```python
from build123d import *

# Parameters (mm, degrees)
BOSS_EXTRUDE1_DEPTH = 2
BOSS_EXTRUDE2_DEPTH = 1
SKETCH3_R           = 3.5
BOSS_EXTRUDE4_DEPTH = 11
SKETCH4_R           = 12.25
BOSS_EXTRUDE5_DEPTH = 6.5


with BuildPart() as part:
    # Sketch1 → Boss-Extrude1 (new body)
    with BuildSketch(Plane(origin=(0, 0, 0), x_dir=(1, 0, 0), z_dir=(0, 1, 0))):
        with BuildLine():
            Line((-14, 10), (-7.665507159, 10))
            ThreePointArc((-7.665507159, 10), (12.6, 0), (-7.665507159, -10))
            Line((-7.665507159, -10), (-14, -10))
            Line((-14, -10), (-14, 10))
        make_face()
    extrude(amount=BOSS_EXTRUDE1_DEPTH)

    # Sketch2 → Boss-Extrude2 (add)
    with BuildSketch(Plane.XY.offset(10)):
        with BuildLine():
            Line((0, 2), (-13.412192981, 19.716181289))
            ThreePointArc((-13.412192981, 19.716181289), (-19.325951381, 20.85226559), (-21.074450498, 15.089802853))
            Line((-21.074450498, 15.089802853), (-14, 0))
            Line((-14, 0), (0, 0))
            Line((0, 0), (0, 2))
        make_face()
    boss_extrude2 = extrude(amount=BOSS_EXTRUDE2_DEPTH)

    # Sketch3 → Boss-Extrude4 (add)
    with BuildSketch(Plane.XY.offset(11)):
        with Locations((-17, 17)):
            Circle(SKETCH3_R)
    boss_extrude4 = extrude(amount=-BOSS_EXTRUDE4_DEPTH)

    # Mirror1: Boss-Extrude2, Boss-Extrude4 across plane
    add(boss_extrude2.mirror(Plane.XY))
    add(boss_extrude4.mirror(Plane.XY))

    # Sketch4 → Boss-Extrude5 (add, symmetric)
    with BuildSketch(Plane.XY):
        with Locations(Location((-17, 17, 0), (0, 0, 180))):
            Circle(SKETCH4_R)
    extrude(amount=BOSS_EXTRUDE5_DEPTH, both=True)


solid = part.part
```
Could you check a few things on this model? Use its own coordinates, in mm. A direction names the side the tool comes from. Coordinates: 2 decimals unless noted, no trailing zeros. Order: outer loops, then holes, each group sorted by start corner. A loop starts at its lowest first (then second) coordinate and runs counter-clockwise, first axis right, second up. Notation, with made-up numbers: M 79.5,-34 L 129.5,-34 A17 ccw 129.5,-26 Z; hole C -32.75,35 d7. An arc over 180 degrees is marked long. Use a Markdown table: item, result. Add a question column.
Q1. I want a section at A-A on z = 0. List the corners of the cut face in (x, y) for me, then the cut area to 3 significant figures.
Q2. Which directions (+Z, -Z, +X, -X, +Y, -Y) give clear straight access to the entire face, cutting with the end or side of a thin tool? Please do faces 1 (the cylindrical face through (-28.684, 13.32, 0.091)), 2 (the flat face through (-17.587, 7.651, -10.493)), 3 (the flat face through (-17.587, 7.651, 10.493)).
Q3. I want a section at C-C on x = -17. List the corners of the cut face in (y, z) for me.
Q4. I want a section at B-B on y = 9. List the corners of the cut face in (x, z) for me, then the cut area to 3 significant figures.
Q5. If I drill on L1, parallel to Z at x = -12, y = 14.75; L2, parallel to Z at x = -6, y = 20.75; L3, parallel to Y at x = 2, z = 10.75, over which ranges is the centre line in solid material (lowest first)?
Q6. I'm going to push flat-ended pins straight in: pin 1 (11 mm diameter, centred on x = -8.5, y = 11.5, fed in from +Z); pin 2 (10 mm diameter, centred on x = -19.5, z = -0.5, fed in from -Y); pin 3 (4 mm diameter, centred on y = 11.5, z = -9, fed in from -X). Where does each tip first touch, or does it pass through?
Q7. We'd pull the mould along Z, two halves only. Please class faces 4 (the flat face through (-14, 1, 0)), 5 (the flat face through (-13, 11, -11)), 6 (the cylindrical face through (12.595, 0.986, -0.367)), 7 (the flat face through (-6.61, 10.73, -10.49)): pulls with the +Z half, pulls with the -Z half, needs draft (parallel to the pull), parting line crosses it, or undercut.
Q8. I want a section at D-D on x = -11. List the corners of the cut face in (y, z) for me.
Checked values:
| question | item | result |
|---|---|---|
| 1 | outline | C -17,17 d24.5; M -14,0 L 12.6,0 L 12.6,2 L -14,2 Z |
| 1 | area | 525 mm² |
| 2 | face 1 | none |
| 2 | face 2 | -Z, -X, -Y |
| 2 | face 3 | +Z, -X, -Y |
| 3 | outline | M 4.75,-6.5 L 13.5,-6.5 L 13.5,-10 L 6.4,-10 L 6.4,-11 L 21.5,-11 L 21.5,-10 L 20.5,-10 L 20.5,-6.5 L 29.25,-6.5 L 29.25,6.5 L 20.5,6.5 L 20.5,10 L 21.5,10 L 21.5,11 L 6.4,11 L 6.4,10 L 13.5,10 L 13.5,6.5 L 4.75,6.5 Z |
| 4 | outline | M -26.28,-6.5 L -7.72,-6.5 L -7.72,6.5 L -26.28,6.5 Z; M -18.22,-11 L -5.3,-11 L -5.3,-10 L -18.22,-10 Z; M -18.22,10 L -5.3,10 L -5.3,11 L -18.22,11 Z |
| 4 | area | 267 mm² |
| 5 | L1 | -11 to -10, -6.5 to 6.5, 10 to 11 |
| 5 | L2 | -6.5 to 6.5 |
| 5 | L3 | 0 to 2 |
| 6 | pin 1 | z = 11 |
| 6 | pin 2 | y = 4.75 |
| 6 | pin 3 | x = -20.2 |
| 7 | face 4 | undercut |
| 7 | face 5 | pulls with the -Z half |
| 7 | face 6 | parting line crosses it |
| 7 | face 7 | needs draft |
| 8 | outline | M 0,-11 L 16.53,-11 L 16.53,-10 L 2,-10 L 2,10 L 16.53,10 L 16.53,11 L 0,11 Z; M 6.32,-6.5 L 27.68,-6.5 L 27.68,6.5 L 6.32,6.5 Z |
